from build123d import *
from build123d.topology import SkipClean

# Parameters (mm, degrees)
SKETCH_1_R           = 4
EXTRUDE_4_DEPTH      = 15
EXTRUDE_5_DEPTH      = 4
SKETCH_15_R          = 5
CUT_EXTRUDE_9_DEPTH  = 118.165082722
SKETCH_16_W          = 16
SKETCH_16_H          = 5
CUT_EXTRUDE_10_DEPTH = 30


with BuildPart() as part:
    # Sketch 1 → Extrude 4 (new, symmetric)
    with BuildSketch(Plane.XY):
        Polygon((0, 0), (40, 0), (40, -12), (80, -12), (80, -4), (118.97114317, 18.5), (114.47114317, 26.294228634), (82.784609691, 8), (0, 8), align=None)
        with Locations((65, -4)):
            Circle(SKETCH_1_R, mode=Mode.SUBTRACT)
    extrude(amount=EXTRUDE_4_DEPTH, both=True)

    # Sketch 1_15 → Extrude 5 (add, symmetric)
    with SkipClean():  # the faces are left unmerged after this step: merging them gives an invalid solid
        with BuildSketch(Plane.XY):
            with BuildLine():
                Line((0, 20), (0, 8))
                Line((0, 8), (65, 8))
                Line((65, 8), (65, 10))
                ThreePointArc((65, 10), (61, 14), (65, 18))
                Line((65, 18), (65, 20))
                Line((65, 20), (0, 20))
            make_face()
            with BuildLine():
                Line((65, 10), (65, 8))
                Line((65, 8), (82.784609691, 8))
                Line((82.784609691, 8), (82.784609691, 20))
                Line((82.784609691, 20), (65, 20))
                Line((65, 20), (65, 18))
                ThreePointArc((65, 18), (67.828427125, 16.828427125), (69, 14))
                ThreePointArc((69, 14), (67.828427125, 11.171572875), (65, 10))
            make_face()
        extrude(amount=EXTRUDE_5_DEPTH, both=True)

    # Sketch 15 → Cut-Extrude 9 (cut, through all)
    with SkipClean():  # the faces are left unmerged after this step: merging them gives an invalid solid
        with BuildSketch(Plane(origin=(17.232050808, -29.846787517, 0), x_dir=(0.8660254037844362, 0.5000000000000044, 0), z_dir=(-0.5000000000000044, 0.8660254037844362, 0))):
            with Locations(Location((102.282032303, 0, 0), (0, 0, 180))):
                Circle(SKETCH_15_R)
        extrude(amount=-CUT_EXTRUDE_9_DEPTH, mode=Mode.SUBTRACT)

    # Sketch 16 → Cut-Extrude 10 (cut)
    with SkipClean():  # the faces are left unmerged after this step: merging them gives an invalid solid
        with BuildSketch(Plane(origin=(97.239092363, 56.141016151, 0), x_dir=(0, 0, -1), z_dir=(0.8660254037844364, 0.5000000000000041, 0))):
            with Locations((0.188244246, -40.964101615)):
                Rectangle(SKETCH_16_W, SKETCH_16_H)
        extrude(amount=-CUT_EXTRUDE_10_DEPTH, mode=Mode.SUBTRACT)


solid = part.part
Read the model definition and answer for the solid it produces. Units are mm, in the model's axes. A direction names the side the tool comes from. Give positions to 0.01 mm unless a question says otherwise; leave off trailing zeros. Write each loop counter-clockwise with the first axis right and the second up, starting at its lowest first coordinate (ties: lowest second). Pieces come first, ordered by that corner, then holes. Notation, with made-up numbers: (8, 8.25) -> (29, 8.25) arc R33 cw to (29, 41.25) -> close; hole circle Ø11 at (86.5, 31.5). An arc over 180 degrees is marked (long way). Answer as a JSON object with one key per item and string values. Group by question number.
1) Find section B-B (x = 77.5). Write down the section's boundary in (y, z), and give its area (3 significant figures).
2) Find section D-D (x = 17). Write down the section's boundary in (y, z).
3) Consider L1, parallel to Y at x = 65, z = 2.5; L2, parallel to Y at x = 65, z = -9; L3, parallel to X at y = 11.5, z = 3. Determine where each line is inside the solid, lowest interval first. Write a range as from..to.
4) A tool of negligible diameter and unlimited length cuts with its end or side. For faces 4 (the flat face through (41, 14, 4)), 5 (the flat face through (82.785, 14, 0)), 6 (the flat face through (100.78, 13.77, -0.08)), from which of +Z, -Z, +X, -X, +Y, -Y can it reach the whole face along a straight path? Write none if from no direction.
5) Each of these flat-tipped pins is pushed along its axis until it touches: P1, Ø1, axis at y = 16.5, z = -4, coming from the +X side; P2, Ø5, axis at x = 30.5, y = 17.5, coming from the +Z side; P3, Ø1.5, axis at x = 31, z = -9.5, coming from the -Y side; P4, Ø12, axis at x = 89.5, y = -7.5, coming from the +Z side. Where does it stop, or does it pass through?
6) Find section A-A (z = -10.75). Write down the section's boundary in (x, y), and give its area (3 significant figures).
7) The mould has two halves that part along Z. Classify faces 1 (the flat face through (59, 3, -15)), 2 (the cylindrical face through (111.123, 22.084, 0.22)), 3 (the flat face through (42, 20, 0)): +Z half, -Z half, draft (parallel to the pull), parting line (faces both ways), or undercut.
8) Find section C-C (z = -1.25). Write down the section's boundary in (x, y), and give its area (3 significant figures).
Values follow:
{
 "1": {"outline": "(-12, -15) -> (8, -15) -> (8, -4) -> (20, -4) -> (20, 4) -> (8, 4) -> (8, 15) -> (-12, 15) -> close", "area": "696 mm2"},
 "2": {"outline": "(0, -15) -> (8, -15) -> (8, -4) -> (20, -4) -> (20, 4) -> (8, 4) -> (8, 15) -> (0, 15) -> close"},
 "3": {"L1": "y = -12..-8, 0..10, 18..20", "L2": "y = -12..-8, 0..8", "L3": "x = 0..61.88, 68.12..82.78, 88.85..96.85"},
 "4": {"face 4": "+Z, -X, +Y", "face 5": "+Z, -Z, +Y", "face 6": "+X"},
 "5": {"P1": "stops at x = 105.85", "P2": "stops at z = 4", "P3": "stops at y = 0", "P4": "passes through"},
 "6": {"outline": "(0, 0) -> (40, 0) -> (40, -12) -> (80, -12) -> (80, -4) -> (118.97, 18.5) -> (114.47, 26.29) -> (82.78, 8) -> (0, 8) -> close; hole circle Ø8 at (65, -4)", "area": "1,450 mm2"},
 "7": {"face 1": "-Z half", "face 2": "undercut", "face 3": "draft"},
 "8": {"outline": "(0, 0) -> (40, 0) -> (40, -12) -> (80, -12) -> (80, -4) -> (92.99, 3.5) -> (90.49, 7.83) -> (103.62, 15.41) -> (101.62, 18.87) -> (82.78, 8) -> (82.78, 20) -> (0, 20) -> close; (110, 23.71) -> (112, 20.25) -> (116.47, 22.83) -> (114.47, 26.29) -> close; hole circle Ø8 at (65, -4); hole circle Ø8 at (65, 14)", "area": "2,210 mm2"}
}
